from build123d import *

# Parameters (mm, degrees)
BOSS_EXTRUDE2_DEPTH     = 45
CUT_EXTRUDE2_DEPTH      = 12
CUT_EXTRUDE4_START      = -33
CUT_EXTRUDE4_DEPTH      = 12
CUT_EXTRUDE5_DEPTH      = 182.957313627
CUT_EXTRUDE7_DEPTH      = 182.957313627
CUT_EXTRUDE7_DEPTH_BACK = 182.957313627


with BuildPart() as part:
    # Sketch1 → Boss-Extrude2 (new body)
    with BuildSketch(Plane(origin=(0, 0, 0), x_dir=(0, 0, -1), z_dir=(1, 0, 0))):
        with BuildLine():
            Line((-59.671894671, -56.645246646), (-25.980762114, -115))
            ThreePointArc((-25.980762114, -115), (0, -130), (25.980762114, -115))
            Line((25.980762114, -115), (59.671894671, -56.645246646))
            ThreePointArc((59.671894671, -56.645246646), (60.926089247, -50.339984724), (58.082708445, -44.574178834))
            Line((58.082708445, -44.574178834), (51.508529611, -38))
            Line((51.508529611, -38), (-51.508529611, -38))
            Line((-51.508529611, -38), (-58.082708445, -44.574178834))
            ThreePointArc((-58.082708445, -44.574178834), (-60.926089247, -50.339984724), (-59.671894671, -56.645246646))
        make_face()
        with BuildLine():
            Line((-23.090724242, -9.582194632), (-51.508529611, -38))
            Line((-51.508529611, -38), (51.508529611, -38))
            Line((51.508529611, -38), (23.090724242, -9.582194632))
            ThreePointArc((23.090724242, -9.582194632), (0, 25), (-23.090724242, -9.582194632))
        make_face()
    extrude(amount=-BOSS_EXTRUDE2_DEPTH)

    # Sketch3 → Cut-Extrude2 (cut)
    with BuildSketch(Plane(origin=(0, 0, 0), x_dir=(0, 0, -1), z_dir=(1, 0, 0))):
        with BuildLine():
            Line((-23.090724242, -9.582194632), (23.090724242, -9.582194632))
            ThreePointArc((23.090724242, -9.582194632), (0, 25), (-23.090724242, -9.582194632))
        make_face()
    extrude(amount=-CUT_EXTRUDE2_DEPTH, mode=Mode.SUBTRACT)

    # Sketch4 → Cut-Extrude4 (cut)
    with BuildSketch(Plane(origin=(0, 0, 0), x_dir=(0, 0, -1), z_dir=(1, 0, 0)).offset(CUT_EXTRUDE4_START)):
        with BuildLine():
            Line((-23.090724242, -9.582194632), (23.090724242, -9.582194632))
            ThreePointArc((23.090724242, -9.582194632), (0, 25), (-23.090724242, -9.582194632))
        make_face()
    extrude(amount=-CUT_EXTRUDE4_DEPTH, mode=Mode.SUBTRACT)

    # Sketch11 → Cut-Extrude5 (cut, through all)
    with BuildSketch(Plane.XY.offset(58.082708445)):
        with BuildLine():
            Line((-12, -9.582194632), (0, -9.582194632))
            Line((0, -9.582194632), (0, -38.192729996))
            ThreePointArc((0, -38.192729996), (-10.975035155, -25.97412099), (-12, -9.582194632))
        make_face()
        with BuildLine():
            Line((-45, -9.582194632), (-33, -9.582194632))
            ThreePointArc((-33, -9.582194632), (-34.024964845, -25.97412099), (-45, -38.192729996))
            Line((-45, -38.192729996), (-45, -9.582194632))
        make_face()
    extrude(amount=-CUT_EXTRUDE5_DEPTH, mode=Mode.SUBTRACT)

    # Sketch12 → Cut-Extrude7 (cut, two sides: drawn at the far end of the back side and taken through both)
    with BuildSketch(Plane.XY.offset(58.082708445).offset(-CUT_EXTRUDE7_DEPTH_BACK)):
        with BuildLine():
            Line((-35, -130.192729996), (-10, -130.192729996))
            Line((-10, -130.192729996), (-10, -48.192729996))
            ThreePointArc((-10, -48.192729996), (-12.928932188, -41.121662184), (-20, -38.192729996))
            Line((-20, -38.192729996), (-25, -38.192729996))
            ThreePointArc((-25, -38.192729996), (-32.071067812, -41.121662184), (-35, -48.192729996))
            Line((-35, -48.192729996), (-35, -130.192729996))
        make_face()
    extrude(amount=CUT_EXTRUDE7_DEPTH + CUT_EXTRUDE7_DEPTH_BACK, mode=Mode.SUBTRACT)


solid = part.part
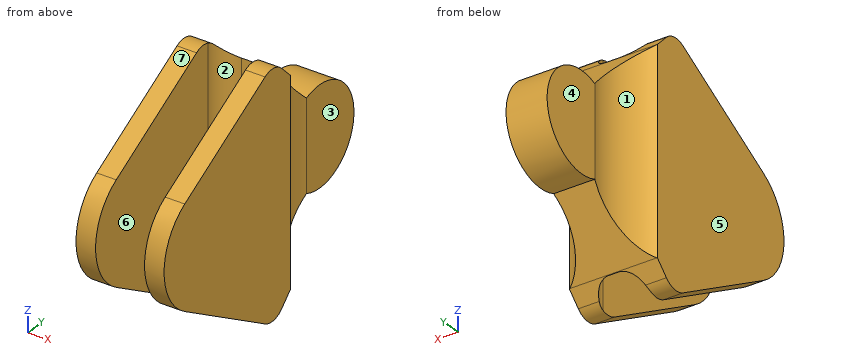
Here's how the part is built. I have some questions about the finished solid (model axes, mm). Face numbers are marked on the shaded views. A direction names the side the tool comes from. Round coordinates to 2 decimals unless told otherwise and drop trailing zeros. Loops run counter-clockwise (first coordinate to the right, second up) from the corner with the lowest first, then second, coordinate; pieces in that order, holes last. Notation, with made-up numbers: (10.25, 58) -> (67.25, 58) arc R31 cw to (67.25, 86) -> close; hole circle Ø9 at (11.25, 64). An arc over 180 degrees is marked (long way). Write each question's results on one line, items separated by ' | '.
(1) If we section it at A-A, the plane y = -95.5: List the corners of the cut face in (x, z) for me.
Worked answers:
outline: (-45, -37.24) -> (-35, -37.24) -> (-35, 37.24) -> (-45, 37.24) -> close; (-10, -37.24) -> (0, -37.24) -> (0, 37.24) -> (-10, 37.24) -> close
(2) If I drill on L1, parallel to X at y = -77.5, z = -14; L2, parallel to X at y = 1, z = 6.5; L3, parallel to Z at x = -2, y = -38, over which ranges is the centre line in solid material (lowest first)?
Worked answers:
L1: -45 to -35, -10 to 0 | L2: -33 to -12 | L3: -51.51 to 51.51
(3) If we section it at D-D, the plane y = 0: List the corners of the cut face in (x, z) for me, then the cut area to 3 significant figures.
Worked answers:
outline: (-33, -25) -> (-12, -25) -> (-12, 25) -> (-33, 25) -> close | area: 1,050 mm2
(4) For the marked faces 1, 2, 3 and 4, which set-ups out of +Z, -Z, +X, -X, +Y, -Y let a thin tool reach every point of the face, with its end or its side?
Worked answers:
face 1: +Z, -Z, -X | face 2: +Z, -Z, -Y | face 3: +Z, -Z, +X, +Y | face 4: +Z, -Z, -X, +Y
(5) We'd pull the mould along X, two halves only. Please class the marked faces 5, 6 and 7: released by +X, released by -X, zero draft, split by the parting line, or undercut.
Worked answers:
face 5: released by -X | face 6: undercut | face 7: zero draft
(6) For P1, Ø2.5, axis at x = -23.5, z = -3, coming from the -Y side; P2, Ø10, axis at x = -14.5, z = -44.5, coming from the +Y side; P3, Ø10.5, axis at y = 11, z = -3, coming from the +X side, each with a flat end and sliding along its axis, tell me the tip position at first contact or that it passes through.
Worked answers:
P1: y = -38.19 | P2: y = -25.99 | P3: x = -12
(7) If we section it at C-C, the plane x = -8: List the corners of the cut face in (y, z) for me, then the cut area to 3 significant figures.
Worked answers:
outline: (-115, -25.98) -> (-56.65, -59.67) arc R10 ccw to (-44.57, -58.08) -> (-31.2, -44.71) -> (-31.2, 44.71) -> (-44.57, 58.08) arc R10 ccw to (-56.65, 59.67) -> (-115, 25.98) arc R30 ccw to start | area: 8,380 mm2
(8) If we section it at B-B, the plane z = 0: List the corners of the cut face in (x, y) for me, then the cut area to 3 significant figures.
Worked answers:
outline: (-45, -130) -> (-35, -130) -> (-35, -48.19) arc R10 cw to (-25, -38.19) -> (-20, -38.19) arc R10 cw to (-10, -48.19) -> (-10, -130) -> (0, -130) -> (0, -38.19) arc R25 cw to (-12, -9.58) -> (-12, 25) -> (-33, 25) -> (-33, -9.58) arc R25 cw to (-45, -38.19) -> close | area: 3,320 mm2
